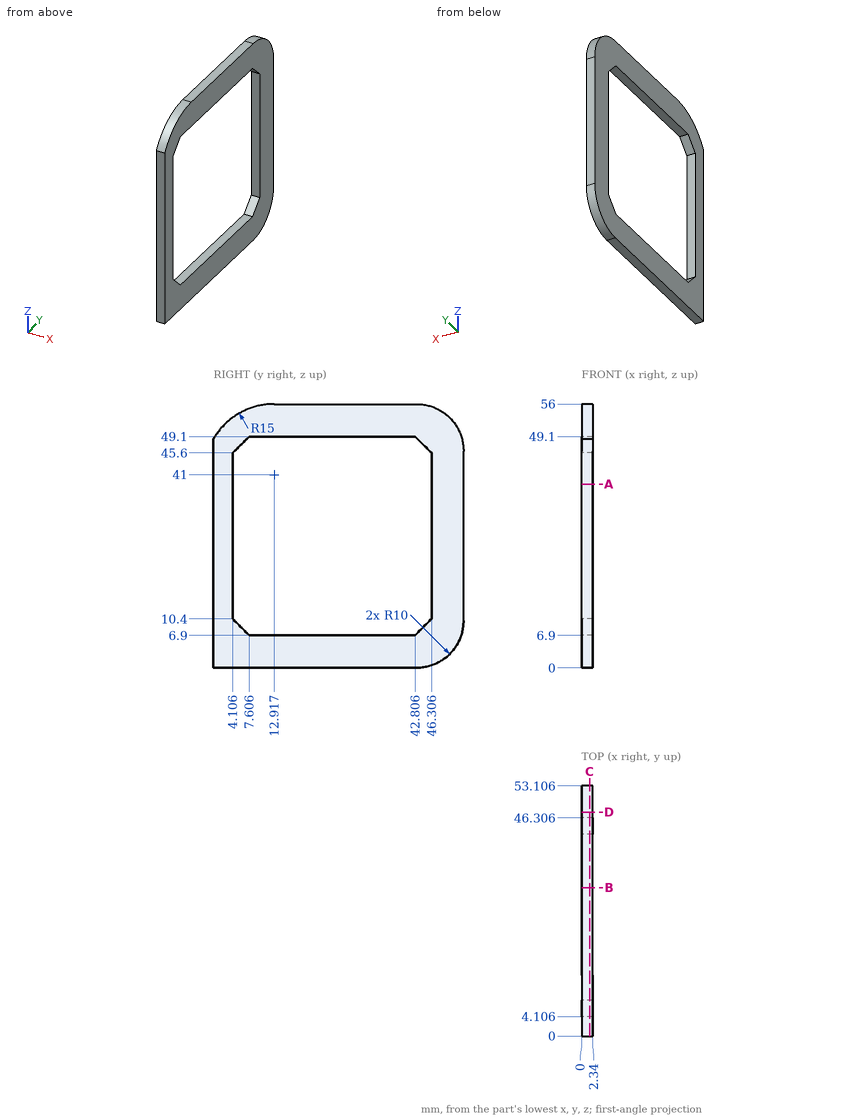
The figure shows three views and two pictorial views of one solid part (mm, origin at its lowest corner). Answer the questions. Coordinates: 2 decimals unless noted, no trailing zeros. Write each loop counter-clockwise with the first axis right and the second up, starting at its lowest first coordinate (ties: lowest second). Pieces come first, ordered by that corner, then holes. Notation, with made-up numbers: (-30, -16) -> (-13, -16) arc R37 ccw to (-13, 22) -> close; hole circle Ø11 at (-6.5, 4). An arc over 180 degrees is marked (long way). Answer as a JSON object with one key per item and string values.
Q1. The part is cut by section D-D on y = 47.5. Give the vertices of the cut face in (x, z), then the cut area to 3 significant figures.
The answers:
{"outline": "(0, 1.02) -> (2.34, 1.02) -> (2.34, 54.98) -> (0, 54.98) -> close", "area": "126 mm2"}
Q2. The part is cut by section C-C on x = 1.7. Give the vertices of the cut face in (y, z).
The answers:
{"outline": "(0, 0) -> (43.11, 0) arc R10 ccw to (53.11, 10) -> (53.11, 46) arc R10 ccw to (43.11, 56) -> (12.92, 56) arc R15 ccw to (0, 48.63) -> close; hole (4.11, 10.4) -> (7.61, 6.9) -> (42.81, 6.9) -> (46.31, 10.4) -> (46.31, 45.6) -> (42.81, 49.1) -> (7.61, 49.1) -> (4.11, 45.6) -> close"}
Q3. The part is cut by section B-B on y = 31.5. Give the vertices of the cut face in (x, z).
The answers:
{"outline": "(0, 0) -> (2.34, 0) -> (2.34, 6.9) -> (0, 6.9) -> close; (0, 49.1) -> (2.34, 49.1) -> (2.34, 56) -> (0, 56) -> close"}
Q4. The part is cut by section A-A on z = 39. Give the vertices of the cut face in (x, y), then the cut area to 3 significant figures.
The answers:
{"outline": "(0, 0) -> (2.34, 0) -> (2.34, 4.11) -> (0, 4.11) -> close; (0, 46.31) -> (2.34, 46.31) -> (2.34, 53.11) -> (0, 53.11) -> close", "area": "25.5 mm2"}
Q5. Consider line 1 (Z direction, x = 1.4, y = 29.5); line 2 (Y direction, x = 1.4, z = 34); line 3 (Z direction, x = 2.15, y = 11.5). Determine where each line is inside the solid, lowest interval first. Write a range as [from, to].
The answers:
{"line 1": "z = [0, 6.9], [49.1, 56]", "line 2": "y = [0, 4.11], [46.31, 53.11]", "line 3": "z = [0, 6.9], [49.1, 55.93]"}
Q6. A flat-ended cylindrical pin translates along its axis: pin 1 Ø2 at (y, z) = (22.5, 9) entering from +X. Find the tip coordinate at first contact, or state that the pin passes through.
The answers:
{"pin 1": "passes through"}
